```python
from build123d import *

# Parameters (mm, degrees)
SKETCH2_R           = 1.5875
SKETCH3_R           = 3.175
BOSS_EXTRUDE1_DEPTH = 19.05
SKETCH4_R           = 2.286
BOSS_EXTRUDE2_DEPTH = 6.35
CHAMFER1_SIZE       = 1.27
CHAMFER1_SIZE2      = 9.525
SKETCH5_W           = 47.5
SKETCH5_H           = 75.5
BOSS_EXTRUDE3_DEPTH = 16
SKETCH6_W           = 8
SKETCH6_H           = 1.5
BOSS_EXTRUDE4_DEPTH = 15.88
DRAFT1_ANGLE        = -5
DRAFT2_ANGLE        = -3
FILLET1_R           = 2.54
FILLET2_R           = 2.54


with BuildPart() as part:
    # Sweep1: sweep along a path in Sketch1
    with BuildLine(Plane.XY) as sweep1_path:
        Line((0, 0), (-101.6, 0))
        ThreePointArc((-101.6, 0), (-128.540768363, 11.159231637), (-139.7, 38.1))
        Line((-139.7, 38.1), (-139.7, 355.6))
    # Sketch2 → Sweep1 (sweep)
    with BuildSketch(Plane(origin=(0, 0, 0), x_dir=(0, 0, -1), z_dir=(1, 0, 0))):
        Circle(SKETCH2_R)
    sweep(path=sweep1_path.line)

    # Sketch3 → Boss-Extrude1 (add)
    with BuildSketch(Plane(origin=(0, 0, 0), x_dir=(0, 0, -1), z_dir=(1, 0, 0))):
        Circle(SKETCH3_R)
    extrude(amount=-BOSS_EXTRUDE1_DEPTH)

    # Sketch4 → Boss-Extrude2 (add)
    with BuildSketch(Plane(origin=(0, 0, 0), x_dir=(0, 0, -1), z_dir=(1, 0, 0))):
        Circle(SKETCH4_R)
    extrude(amount=BOSS_EXTRUDE2_DEPTH)

    # Chamfer1
    chamfer1_edges = [part.edges().sort_by_distance(p)[0] for p in [
        (-19.05, 0, 3.175),
    ]]
    chamfer1_side = [part.faces().sort_by_distance(p)[0] for p in [
        (-19.05, 0, 3.085197439),
    ]]
    chamfer(chamfer1_edges, length=CHAMFER1_SIZE, length2=CHAMFER1_SIZE2, reference=chamfer1_side[0])

    # Sketch5 → Boss-Extrude3 (add, symmetric)
    with BuildSketch(Plane.XY):
        with Locations((-123.8875, 317.85)):
            Rectangle(SKETCH5_W, SKETCH5_H)
    extrude(amount=BOSS_EXTRUDE3_DEPTH, both=True)

    # Sketch6 → Boss-Extrude4 (add)
    with BuildSketch(Plane(origin=(-147.6375, 0, 0), x_dir=(0, 0, -1), z_dir=(1, 0, 0))):
        with Locations((0, 336.55)):
            Rectangle(SKETCH6_W, SKETCH6_H)
        with Locations((0, 320.04)):
            Rectangle(SKETCH6_W, SKETCH6_H)
    extrude(amount=-BOSS_EXTRUDE4_DEPTH)

    # Draft1
    draft1_faces = [part.faces().sort_by_distance(p)[0] for p in [
        (-123.804705338, 280.1, 0),
        (-123.8875, 355.6, 0),
    ]]
    draft(draft1_faces, Plane(origin=(-147.6375, 355.6, 16), x_dir=(0, 0, -1), z_dir=(-1, 0, 0)), DRAFT1_ANGLE)

    # Draft2
    draft2_faces = [part.faces().sort_by_distance(p)[0] for p in [
        (-124.348635482, 317.85, -16),
        (-124.348635482, 317.85, 16),
    ]]
    draft(draft2_faces, Plane(origin=(-147.6375, 355.6, 16), x_dir=(0, 0, -1), z_dir=(-1, 0, 0)), DRAFT2_ANGLE)

    # Fillet1
    fillet1_edges = [part.edges().sort_by_distance(p)[0] for p in [
        (-123.8875, 353.522144241, -14.755315242),
        (-100.1375, 351.444288483, 0),
        (-123.8875, 282.177855759, -14.755315242),
        (-100.1375, 317.85, -13.510630484),
        (-100.1375, 284.255711517, 0),
        (-100.1375, 317.85, 13.510630484),
        (-123.8875, 353.522144241, 14.755315242),
        (-123.8875, 282.177855759, 14.755315242),
    ]]
    fillet(fillet1_edges, radius=FILLET1_R)

    # Fillet2
    fillet2_edges = [part.edges().sort_by_distance(p)[0] for p in [
        (-163.5175, 336.55, -4),
        (-163.5175, 336.55, 4),
        (-163.5175, 320.04, -4),
        (-163.5175, 320.04, 4),
    ]]
    fillet(fillet2_edges, radius=FILLET2_R)


solid = part.part
```
Part model, mm, in its own coordinate system. A direction names the side the tool comes from. Round coordinates to 2 decimals unless told otherwise and drop trailing zeros. Loops run counter-clockwise (first coordinate to the right, second up) from the corner with the lowest first, then second, coordinate; pieces in that order, holes last.
1. Two-plate mould, pull along Y, no slides. Class faces 1 (the face through (-155, 319.29, 0)), 2 (the face through (-100.138, 317, 0)), 3 (the face through (-155, 335.8, 0)): pulls with the +Y half, pulls with the -Y half, needs draft (parallel to the pull), parting line crosses it, or undercut.
Solutions:
face 1: pulls with the -Y half
face 2: needs draft
face 3: undercut
2. Flat gauge pins, fed straight in: pin 1 (1.6 mm diameter, centred on x = -152.5, y = 336.5, fed in from +Z); pin 2 (12 mm diameter, centred on x = -11.5, z = -8, fed in from +Y); pin 3 (0.8 mm diameter, centred on x = -155, y = 320, fed in from -Z). Where does each tip first touch, or does it go through?
Solutions:
pin 1: stops at z = 4
pin 2: stops at y = 2.22
pin 3: stops at z = -4
3. 3-axis set-ups, long thin cutter, end or side, ignore diameter. For faces 4 (the face through (-14.22, -2.49, 0.55)), 5 (the face through (-155, 337.3, 0)), 6 (the face through (-155, 320.79, 0)), 7 (the face through (0, -2.1, -1.4)), 8 (the face through (-124.73, 282.83, 14.04)): which of +Z, -Z, +X, -X, +Y, -Y reach the whole face in a straight line?
Solutions:
face 4: none
face 5: +Z, -Z, -X, +Y
face 6: +Z, -Z, -X
face 7: +X
face 8: +Z, +X, -Y
4. Drill centre lines: line 1 along X through (y, z) = (306, 4); line 2 along Y through (x, z) = (-60, 0.5); line 3 along Y through (x, z) = (-131, 9.5). Where is each one in solid material? Low to high.
Solutions:
line 1: x = -147.64 to -100.14
line 2: y = -1.51 to 1.51
line 3: y = 281.56 to 354.14
5. Slice it at B-B (x = -56). Give the cut face in (y, z) (1 decimal).
Solutions:
outline: circle Ø3.2 at (0, 0)
6. Slice it at A-A (y = 162.5). Give the cut face in (x, z) (1 decimal).
Solutions:
outline: circle Ø3.2 at (-139.7, 0)
